Input: dimensioned drawing with shaded views. Units: mm. Origin: part minimum x, y, z. A direction names the side the tool comes from. Coordinates: 2 decimals unless noted, no trailing zeros. Order: outer loops, then holes, each group sorted by start corner. A loop starts at its lowest first (then second) coordinate and runs counter-clockwise, first axis right, second up. Notation, with made-up numbers: M 63,-12.5 L 100,-12.5 A29 ccw 100,25.5 Z; hole C 4,66 d3. An arc over 180 degrees is marked long. Write item = value, one per line.
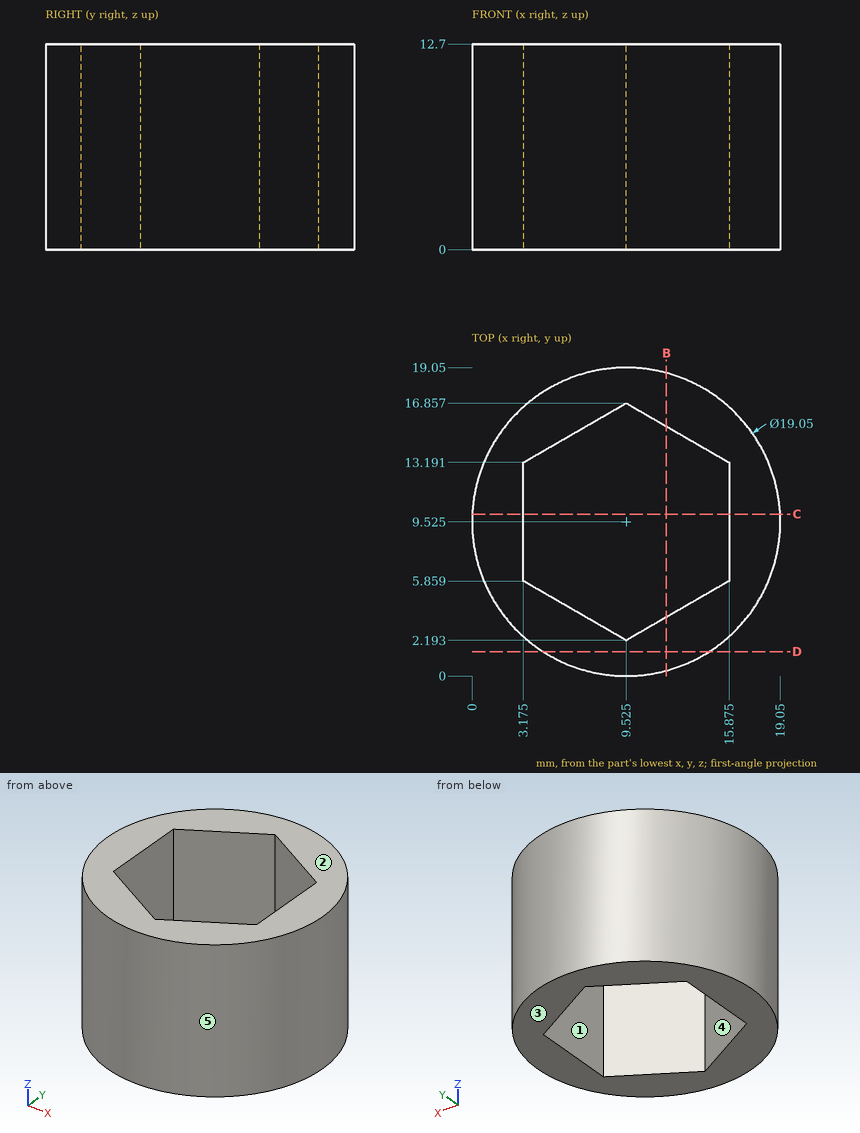
1) Pin query (flat end, axial travel): pin 1 (8 mm diameter, centred on x = 10, y = 10.5, fed in from +Z); pin 2 (6 mm diameter, centred on x = 5, z = 4.5, fed in from -Y); pin 3 (1 mm diameter, centred on y = 15, z = 9.5, fed in from +X); pin 4 (2 mm diameter, centred on x = 16.5, z = 3, fed in from +Y). Return the tip coordinate at first contact, or that it passes through.
Numbers:
pin_1 = through
pin_2 = 0.12
pin_3 = 17.65
pin_4 = 16.94
2) Mould query, pull axis X, two halves, no side actions, for the marked faces 3, 4 and 5. Classes: pulls with the +X half, pulls with the -X half, needs draft (parallel to the pull), parting line crosses it, or undercut.
Numbers:
face_3 = needs draft
face_4 = undercut
face_5 = parting line crosses it
3) Section D-D, the plane y = 1.5. Return loops of the section in (x, z), and give its area (3 significant figures).
Numbers:
outline = M 4.39,0 L 14.66,0 L 14.66,12.7 L 4.39,12.7 Z
area = 130 mm²
4) Line query: L1, parallel to X at y = 9.75, z = 7 (1 decimal); L2, parallel to Y at x = 9.5, z = 10; L3, parallel to Y at x = 4.75, z = 0.5. Output: solid intervals per line, ascending.
Numbers:
L1 = 0 to 3.2, 15.9 to 19
L2 = 0 to 2.21, 16.84 to 19.05
L3 = 1.28 to 4.95, 14.1 to 17.77
5) Set-up query: the marked faces 1 and 2. Return all of +Z, -Z, +X, -X, +Y, -Y with unobstructed straight access to the full face (end or side cutting, diameter ignored); none if empty.
Numbers:
face_1 = +Z, -Z
face_2 = +Z, +X, -X, +Y, -Y
6) Section B-B, the plane x = 12. Return loops of the section in (y, z).
Numbers:
outline = M 0.33,0 L 3.62,0 L 3.62,12.7 L 0.33,12.7 Z; M 15.43,0 L 18.72,0 L 18.72,12.7 L 15.43,12.7 Z
7) Section C-C, the plane y = 10. Return loops of the section in (x, z) (1 decimal).
Numbers:
outline = M 0,0 L 3.2,0 L 3.2,12.7 L 0,12.7 Z; M 15.9,0 L 19,0 L 19,12.7 L 15.9,12.7 Z
